Design review of the part built by this model. Coordinates are the model's own, in mm. Give positions to 0.01 mm unless a question says otherwise; leave off trailing zeros. Loops run counter-clockwise (first coordinate to the right, second up) from the corner with the lowest first, then second, coordinate; pieces in that order, holes last.
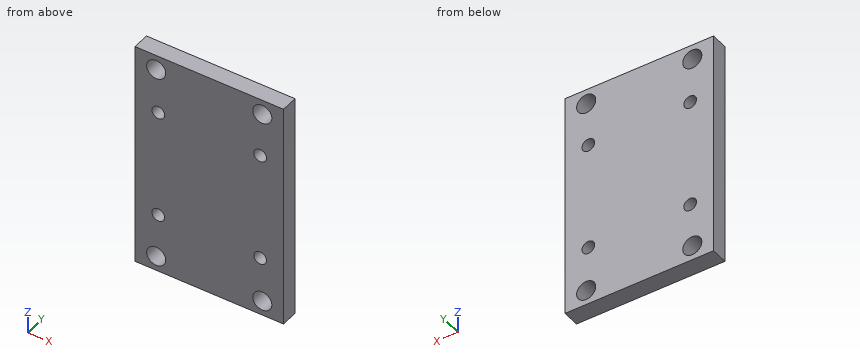
from build123d import *

# Parameters (mm, degrees)
F0_W     = 70
F0_H     = 107
F0_R     = 4.5
F1_DEPTH = 8
F3_D     = 6
F3_DEPTH = 21


with BuildPart() as f1:
    # F0 (on Front) → F1 (new body)
    with BuildSketch(Plane.XZ):
        Rectangle(F0_W, F0_H)
        with Locations((-25, -46.5)):
            Circle(F0_R, mode=Mode.SUBTRACT)
        with Locations((25, -46.5)):
            Circle(F0_R, mode=Mode.SUBTRACT)
        with Locations((-25, 46.5)):
            Circle(F0_R, mode=Mode.SUBTRACT)
        with Locations((25, 46.5)):
            Circle(F0_R, mode=Mode.SUBTRACT)
    extrude(amount=F1_DEPTH)

    # F3
    with Locations(Plane.XZ.offset(8)):
        with Locations((-24, 25.5), (24, 25.5), (-24, -25.5), (24, -25.5)):
            Hole(F3_D / 2, depth=F3_DEPTH)


solid = f1.part
Q1. Take a section at B-B (y = -5). Give the number of separate pieces and of enclosed holes in the cut face, plus the area to 3 significant figures.
Results:
separate pieces: 1
enclosed holes: 8
area: 7,120 mm2
Q2. Wall thickness on line 1 (Z direction, x = 24, y = -2.75); line 2 (Z direction, x = -24.5, y = -7); line 3 (X direction, y = -6.75, z = -27): over which ranges is each line inside the solid? List them lowest first.
Results:
line 1: z = -53.5 to -50.89, -42.11 to -28.5, -22.5 to 22.5, 28.5 to 42.11, 50.89 to 53.5
line 2: z = -53.5 to -50.97, -42.03 to -28.46, -22.54 to 22.54, 28.46 to 42.03, 50.97 to 53.5
line 3: x = -35 to -26.6, -21.4 to 21.4, 26.6 to 35
Q3. Take a section at A-A (z = -46.5). Give the boundary of the cut face in (x, y), plus the area to 3 significant figures.
Results:
outline: (-35, -8) - (-29.5, -8) - (-29.5, 0) - (-35, 0) - close; (-20.5, -8) - (20.5, -8) - (20.5, 0) - (-20.5, 0) - close; (29.5, -8) - (35, -8) - (35, 0) - (29.5, 0) - close
area: 416 mm2
Q4. Take a section at C-C (x = -25). Give the boundary of the cut face in (y, z), plus the area to 3 significant figures.
Results:
outline: (-8, -53.5) - (0, -53.5) - (0, -51) - (-8, -51) - close; (-8, -42) - (0, -42) - (0, -28.33) - (-8, -28.33) - close; (-8, -22.67) - (0, -22.67) - (0, 22.67) - (-8, 22.67) - close; (-8, 28.33) - (0, 28.33) - (0, 42) - (-8, 42) - close; (-8, 51) - (0, 51) - (0, 53.5) - (-8, 53.5) - close
area: 621 mm2
Q5. Take a section at D-D (z = 25.5). Give the boundary of the cut face in (x, y).
Results:
outline: (-35, -8) - (-27, -8) - (-27, 0) - (-35, 0) - close; (-21, -8) - (21, -8) - (21, 0) - (-21, 0) - close; (27, -8) - (35, -8) - (35, 0) - (27, 0) - close
Q6. Insertion check: pin 1 (8 mm diameter, centred on x = 25, z = 46.5, fed in from -Y). The pin has a flat end and moves straight along its axis. Give the tip position at first contact, or say it passes through.
Results:
pin 1: passes through
